Check sheet for the modelled part. Datum: model origin and axes. Units: mm. A direction names the side the tool comes from. Round coordinates to 2 decimals unless told otherwise and drop trailing zeros. Loops run counter-clockwise (first coordinate to the right, second up) from the corner with the lowest first, then second, coordinate; pieces in that order, holes last. Notation, with made-up numbers: (38, -26) -> (59, -26) arc R13 ccw to (59, -7) -> close; hole circle Ø7 at (57.25, 12.5). An arc over 180 degrees is marked (long way). Use one line per item in the form item = value. Start each with the question number.
(1) Sectioned sample at B-B (x = 7.25). Record the cut outline in (y, z), and give its area (3 significant figures).
(2) Draft check along Z on faces 1 (the flat face through (0, 0, 2)), 2 (the flat face through (1.121, -0.761, -1.293)), 3 (the cylindrical face through (5.27, -0.54, 2.44)). Enter one of: released by +Z, released by -Z, zero draft, split by the parting line, or undercut.
(3) Set-up check for faces 4 (the flat face through (1.121, 0.761, 1.293)), 5 (the cylindrical face through (0.449, -0.614, 4.675)): record each of +Z, -Z, +X, -X, +Y, -Y from which the full face is reachable in a straight line by a thin tool's end or side.
(4) Go/stop test with flat-tipped pins: pin 1 (1.5 mm diameter, centred on y = 1, z = 2, fed in from +X); pin 2 (1.4 mm diameter, centred on x = 1.5, z = 0.5, fed in from -Y); pin 3 (3 mm diameter, centred on x = 2, y = 3, fed in from +Z); pin 4 (2 mm diameter, centred on x = 1.5, y = -1.5, fed in from -Z). Record where each tip stops, or that it passes through.
(5) Sectioned sample at A-A (x = 0.5). Record the cut outline in (y, z) (3 decimals).
(6) Material ranges on probe 1 along Z at (x, y) = (1.75, 0.75); probe 2 along Y at (x, z) = (1.5, 0.5); probe 3 along Y at (x, z) = (3.5, -2), recorded low to high. Write a range as [from, to].
Autodesk Inventor part; units mm, degrees
ref_plane "Work Plane1" through (104.775, 0, 0) normal (0, 0, -1) x (1, 0, 0)
ref_plane "YZ Plane" through (0, 0, 0) normal (1, 0, 0) x (0, 1, 0)
ref_plane "XZ Plane" through (0, 0, 0) normal (0, 1, 0) x (-1, 0, 0)
sketch "Esquisse1" plane through (0, 0, 0) normal (0, 0, 1) x (1, 0, 0)
  line L0 (8, 0) -> (8, 2.5)
  line L1 (8, 2.5) -> (5.6, 2.5)
  line L2 (5.6, 2.5) -> (5.1092, 2.5)
  line L3 (0, 4.715) -> (0, 1.7321)
  line L4 (0, 1.7321) -> (2.14, 1.7321)
  line L5 (2.14, 1.7321) -> (3.14, 0)
  line L6 (3.14, 0) -> (8, 0)
  line L7 (0, 4.715) -> (0.885, 4.715)
  line L8 (0.885, 4.715) -> (3.1, 2.5)
  line L9 (5.1092, 2.5) -> (3.1, 2.5)
  line L10 (5.6, 2.5) -> (3.1, 2.5) construction
  line L11 (3.1, 2.5) -> (3.1, 2.5)
  line L12 (-1.6, 0) -> (9.6, 0)
  line L13 (0, -0.943) -> (0, 5.658)
  dimension "d0" = 8
  dimension "d1" = 2.4
  dimension "d2" = 2.14
  dimension "d3" = 5
  dimension "d6" = 3.1
  dimension "d7" = 45
  dimension "d8" = 3.4641
  dimension "d9" = 60
  dimension "d10" = 9.43
  dimension "d11" = 5
  dimension "d12" = 0.4908
revolve "Corps" add sketch "Esquisse1" angle 360 about axis through (3.14, 0, 0) along (1, 0, 0) contours L6 L5 L4 L3 L7 L8 L9 L2 L1 L0
sketch "Esquisse2" plane through (0, 0, 0) normal (-1, 0, 0) x (0, 0, 1)
  circle A0 centre (0, 0) radius 1.7321
  line L0 (0, -6.601) -> (0, 6.601)
  line L1 (-6.601, 0) -> (6.601, 0)
  line L2 (1.7321, 0) -> (0.866, -1.5)
  line L3 (0.866, -1.5) -> (-0.866, -1.5)
  line L4 (-0.866, -1.5) -> (-1.7321, 0)
  line L5 (-1.7321, 0) -> (-0.866, 1.5)
  line L6 (-0.866, 1.5) -> (0.866, 1.5)
  line L7 (0.866, 1.5) -> (1.7321, 0)
  point P0 (0, 1.7321)
extrude "Rainure" add sketch "Esquisse2" against normal up to next contours L7 A0 | A0 L2 | L6 L0 A0 | A0 L0 L3 | L0 L6 A0 | A0 L3 L0 | L4 A0 | A0 L5
thread "Filetage"
chamfer "Chanfrein1" distance 0.4908 distance2 0.4908 1 edges at (8, -2.5, 0) measured on face at (8, 0.4809, 1.5312)
ref_plane "Work Plane1" through (104.775, 0, 0) normal (0, 0, -1) x (1, 0, 0)
equation "\"d15\" = GEL"
equation "\"d17\" = -0.5 * SPD + 0.5 * GD"
equation "\"d18\" = GUL"
equation "\"d0\" = NLG"
equation "\"d1\" = GEL"
equation "\"d2\" = INTI"
equation "\"d3\" = GD"
equation "\"d6\" = KOH"
equation "\"d7\" = 0.5 * SEWI"
equation "\"d8\" = 1.1547 * SW"
equation "\"d10\" = KOD"
equation "\"d11\" = BDM"
equation "\"d12\" = GAL"
equation "\"NLG\" = 8"
equation "\"INTI\" = 2.14"
equation "\"GEL\" = 2.4"
equation "\"GAL\" = 0.61345 * PTC"
equation "\"KOH\" = 3.1"
equation "\"KOD\" = 9.43"
equation "\"GUL\" = 0.61345 * PTC"
equation "\"SPD\" = NND - 1.2269 * PTC"
equation "\"BDM\" = NND"
equation "\"GD\" = NND"
equation "\"SEWI\" = 90deg"
equation "\"SW\" = 3"
equation "\"TOA\" = 30deg"
equation "\"GD1\" = THREADDIA - 1.2269 * PTC"
equation "\"EPV\" = 5.6"
equation "\"THREADDIA\" = 5"
equation "\"PTC\" = 0.8"
equation "\"NND\" = 5"
equation "\"E0\" = 3.47"
equation "\"THREADDESC\" = 1.2345"
properties part number "ISO 10642 - M5 x  8" material "Acier"
Checks:
q1.outline = circle Ø5 at (0, 0)
q1.area = 19.6 mm2
q2.face_1 = zero draft
q2.face_2 = undercut
q2.face_3 = split by the parting line
q3.face_4 = -X
q3.face_5 = +X, -X
q4.pin_1 = 8
q4.pin_2 = -4.71
q4.pin_3 = 4.27
q4.pin_4 = -4.66
q5.outline = circle Ø9.43 at (0, 0); hole (-1.5, -0.866) -> (0, -1.732) -> (1.5, -0.866) -> (1.5, 0.866) -> (0, 1.732) -> (-1.5, 0.866) -> close
q6.probe_1 = [-3.78, -1.3], [1.3, 3.78]
q6.probe_2 = [-4.07, -1.5], [1.5, 4.07]
q6.probe_3 = [-1.5, 1.5]
